Autodesk Inventor part; units mm, degrees
ref_plane "YZ Plane" through (0, 0, 0) normal (1, 0, 0) x (0, 1, 0)
ref_plane "XZ Plane" through (0, 0, 0) normal (0, 1, 0) x (-1, 0, 0)
ref_plane "XY Plane" through (0, 0, 0) normal (0, 0, 1) x (1, 0, 0)
sketch "Sketch1" plane through (0, 0, 0) normal (0, 1, 0) x (-1, 0, 0)
  line L0 (0, 0) -> (25.4, 0)
  line L1 (25.4, 0) -> (25.4, -3.175)
  line L2 (25.4, -3.175) -> (3.175, -3.175)
  line L3 (3.175, -3.175) -> (3.175, -25.4)
  line L4 (3.175, -25.4) -> (0, -25.4)
  line L5 (0, -25.4) -> (0, 0)
  dimension "d0" = 25.4
  dimension "d1" = 3.175
  dimension "d2" = 90
  dimension "d7" = 25.4
  dimension "d8" = 3.175
extrude "Extrusion1" add sketch "Sketch1" along normal blind 511.8354
sketch "Sketch2" plane through (0, 0, 0) normal (1, 0, 0) x (0, 0, -1)
  line L0 (25.4, 0) -> (25.4, 511.8354)
  line L1 (25.4, 511.8354) -> (50.8817, 511.8354) construction
  line L2 (0, 511.8354) -> (25.4, 511.8354)
  line L3 (25.4, 511.8354) -> (0, 509.7962)
  line L4 (0, 0) -> (0, 511.8354)
  line L5 (25.4, 511.8354) -> (50.8817, 511.8354) construction
  line L6 (0, 509.7962) -> (0, 511.8354)
  line L7 (25.4, 511.8354) -> (0, 511.8354)
  line L8 (25.4, 0) -> (0, 0)
  line L9 (0, 0) -> (25.4, 2.0392)
  line L10 (0, 0) -> (25.4817, 0) construction
  line L11 (25.4, 2.0392) -> (25.4, 0)
  line L12 (25.4, 0) -> (0, 0)
  dimension "d10" = 175.41
  dimension "d11" = 4.59
extrude "Extrusion2" cut sketch "Sketch2" against normal through all contours L8 L9 L0 | L3 L4 L2
properties part number "AngleL" material "Aluminum 6061"
Geometry check sheet. Reference: the model listing, model coordinates, mm. A direction names the side the tool comes from. Coordinates: 2 decimals unless noted, no trailing zeros. Order: outer loops, then holes, each group sorted by start corner. A loop starts at its lowest first (then second) coordinate and runs counter-clockwise, first axis right, second up.
Q1. Sectioned sample at B-B on x = -11. Record the cut outline in (y, z) (3 decimals), and give its area (3 significant figures).
Reply:
outline: (0, 0) - (0.255, -3.175) - (510.051, -3.175) - (509.796, 0) - close
area: 1,620 mm2
Q2. Thickness scan on probe 1 along Z at (x, y) = (-7, 280) (3 decimals); probe 2 along Y at (x, z) = (-2.25, -4.5). Record the ranges inside material, lowest first.
Reply:
probe 1: z = -3.175 to 0
probe 2: y = 0.36 to 510.16
Q3. Sectioned sample at A-A on y = 111.5. Record the cut outline in (x, z) (3 decimals).
Reply:
outline: (-25.4, -3.175) - (-3.175, -3.175) - (-3.175, -25.4) - (0, -25.4) - (0, 0) - (-25.4, 0) - close
Q4. Tool access check on faces 1 (the face through (-3.175, 252, -14)), 2 (the face through (-2.293, 510.443, -8.056)). Record the directions out of +Z, -Z, +X, -X, +Y, -Y that give a thin tool (end or side, any length) a straight path to the whole face; none if there is none.
Reply:
face 1: -Z, -X, +Y, -Y
face 2: +Z, +X, -X, +Y
Q5. Depth check by flat-ended pin: pin 1 Ø2 at (x, z) = (-3.5, -16.5) entering from -Y; pin 2 Ø1.5 at (x, y) = (-10.5, 263.5) entering from -Z (3 decimals); pin 3 Ø1.5 at (y, z) = (136.5, -4.5) entering from -X (3 decimals). Enter the tip coordinate at first touch or a pass-through.
Reply:
pin 1: stops at y = 1.25
pin 2: stops at z = -3.175
pin 3: stops at x = -3.175
Q6. Sectioned sample at C-C on z = -16. Record the cut outline in (x, y) (3 decimals).
Reply:
outline: (-3.175, 1.285) - (0, 1.285) - (0, 511.081) - (-3.175, 511.081) - close
